The figure shows three views and two pictorial views of one solid part (mm, origin at its lowest corner). Answer the questions. A direction names the side the tool comes from. Give positions to 0.01 mm unless a question says otherwise; leave off trailing zeros. Loops run counter-clockwise (first coordinate to the right, second up) from the corner with the lowest first, then second, coordinate; pieces in that order, holes last. Notation, with made-up numbers: M -3.5,81.5 L 55.5,81.5 A30 ccw 55.5,114.5 Z; hole C 59.5,74.25 d1. An arc over 180 degrees is marked long. One line per item, written item: value. Start each with the question number.
Q1. A cutting plane is placed at A-A, the plane y = 37.5. Determine the outline of the cut face in (x, z).
Q2. A cutting plane is placed at B-B, the plane x = 5. Determine the outline of the cut face in (y, z), and give its area (3 significant figures).
Q3. The mould has two halves that part along X. Classify the marked faces 5, 6, 7 and 8: +X half, -X half, draft (parallel to the pull), parting line (faces both ways), or undercut.
Q4. A cutting plane is placed at C-C, the plane z = 5. Determine the outline of the cut face in (x, y).
Q5. Consider L1, parallel to Z at x = 8.2, y = 37.5; L2, parallel to X at y = 38.5, z = 8.5; L3, parallel to X at y = 37.5, z = 2.25. Determine where each line is inside the solid, lowest interval first.
Q6. For the marked faces 1, 2, 3 and 4, determine the directions among +Z, -Z, +X, -X, +Y, -Y from which every point of the face is accessible in a straight line to the end or side of a thin tool.
Q7. Flat-ended cylindrical pins translate along their axes: pin 1 (4.5 mm diameter, centred on y = 2, z = 7.5, fed in from +X); pin 2 (1.2 mm diameter, centred on y = 1, z = 6.5, fed in from -X). Find the tip coordinate at first contact, or state that the pin passes through.
Q8. A cutting plane is placed at D-D, the plane z = 3. Determine the outline of the cut face in (x, y), and give its area (3 significant figures).
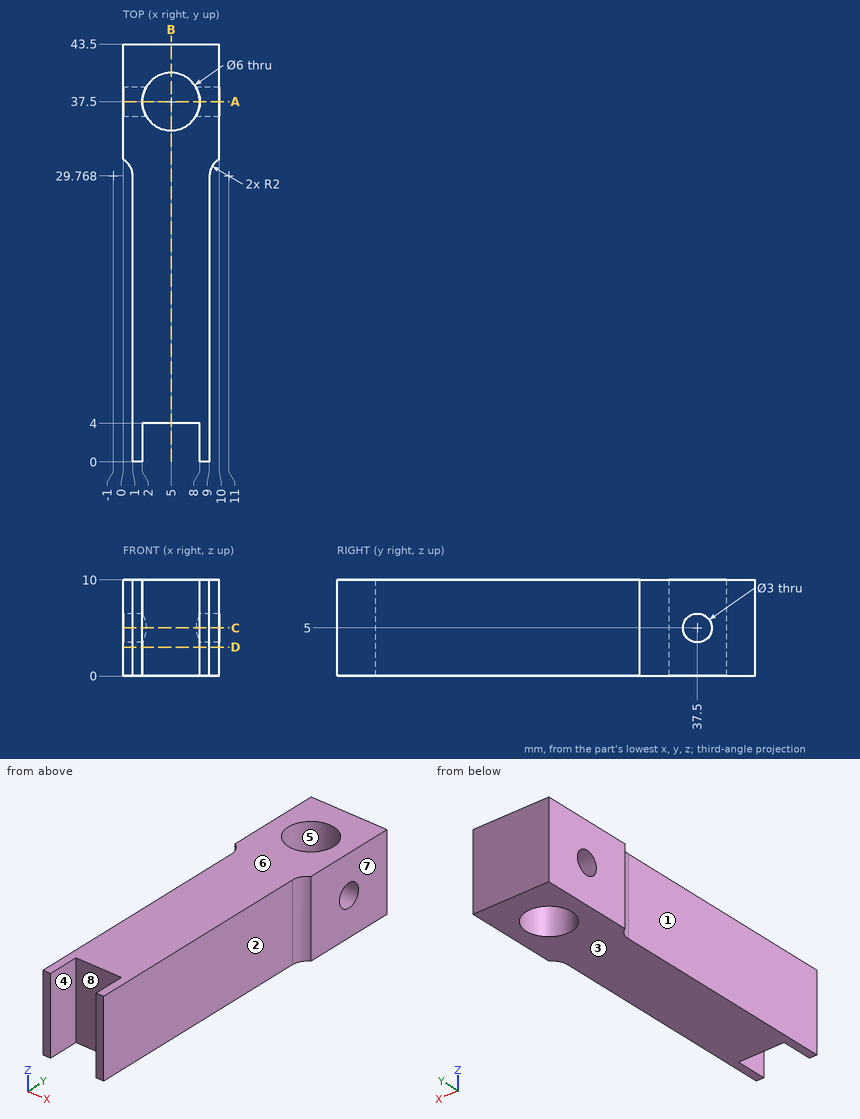
Answer block:
1. outline: M 0,0 L 2,0 L 2,3.5 L 0,3.5 Z; M 0,6.5 L 2,6.5 L 2,10 L 0,10 Z; M 8,0 L 10,0 L 10,3.5 L 8,3.5 Z; M 8,6.5 L 10,6.5 L 10,10 L 8,10 Z
2. outline: M 4,0 L 34.5,0 L 34.5,10 L 4,10 Z; M 40.5,0 L 43.5,0 L 43.5,10 L 40.5,10 Z
2. area: 335 mm^2
3. face 5: undercut
3. face 6: draft
3. face 7: +X half
3. face 8: undercut
4. outline: M 0,31.5 A2 cw 1,29.77 L 1,0 L 2,0 L 2,4 L 8,4 L 8,0 L 9,0 L 9,29.77 A2 cw 10,31.5 L 10,36 L 7.6,36 A3 cw 2.4,36 L 0,36 Z; M 0,39 L 2.4,39 A3 cw 7.6,39 L 10,39 L 10,43.5 L 0,43.5 Z
5. L1: 0 to 3.5, 6.5 to 10
5. L2: 0 to 2.17, 7.83 to 10
5. L3: 0 to 2, 8 to 10
6. face 1: +Z, -Z, -X, -Y
6. face 2: +Z, -Z, +X, -Y
6. face 3: -Z, +X, -X, +Y, -Y
6. face 4: +Z, -Z, -Y
7. pin 1: x = 9
7. pin 2: x = 1
8. outline: M 0,31.5 A2 cw 1,29.77 L 1,0 L 2,0 L 2,4 L 8,4 L 8,0 L 9,0 L 9,29.77 A2 cw 10,31.5 L 10,43.5 L 0,43.5 Z; hole C 5,37.5 d6
8. area: 321 mm^2
